Could you check a few things on this model? Use its own coordinates, in mm. Face numbers are marked on the shaded views. A direction names the side the tool comes from. Give positions to 0.01 mm unless a question says otherwise; leave off trailing zeros. Order: outer loops, then holes, each group sorted by start corner. A loop starts at its lowest first (then second) coordinate and runs counter-clockwise, first axis right, second up.
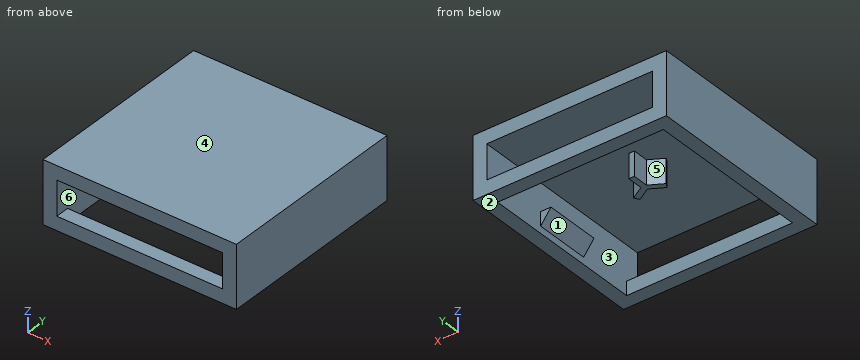
from build123d import *

# Parameters (mm, degrees)
SKETCH_1_W          = 28
SKETCH_1_H          = 28
EXTRUDE_1_DEPTH     = 2
SKETCH_2_W          = 28
SKETCH_2_H          = 28
SKETCH_2_W_2        = 24
SKETCH_2_H_2        = 24
EXTRUDE_2_DEPTH     = 7
SKETCH_3_W          = 24
SKETCH_3_H          = 5
CUT_EXTRUDE_1_DEPTH = 33.078029865
EXTRUDE_3_DEPTH     = 3.5
EXTRUDE_4_DEPTH     = 4


with BuildPart() as part:
    # Эскиз1 → Бобышка-Вытянуть1 (new body)
    with BuildSketch(Plane.XY):
        Rectangle(SKETCH_1_W, SKETCH_1_H)
    extrude(amount=EXTRUDE_1_DEPTH)

    # Эскиз2 → Бобышка-Вытянуть2 (add)
    with BuildSketch(Plane(origin=(0, 0, 0), x_dir=(-1, 0, 0), z_dir=(0, 0, -1))):
        Rectangle(SKETCH_2_W, SKETCH_2_H)
        Rectangle(SKETCH_2_W_2, SKETCH_2_H_2, mode=Mode.SUBTRACT)
    extrude(amount=EXTRUDE_2_DEPTH)

    # Эскиз3 → Вырез-Вытянуть1 (cut, through all)
    with BuildSketch(Plane(origin=(0, 14, 0), x_dir=(1, 0, 0), z_dir=(0, 1, 0))):
        with Locations((0, 2.5)):
            Rectangle(SKETCH_3_W, SKETCH_3_H)
    extrude(amount=-CUT_EXTRUDE_1_DEPTH, mode=Mode.SUBTRACT)

    # Эскиз4 → Бобышка-Вытянуть3 (add)
    with BuildSketch(Plane(origin=(0, 0, 0), x_dir=(-1, 0, 0), z_dir=(0, 0, -1))):
        with BuildLine():
            Line((-1.965063509, -1.596410162), (0, -0.461880215))
            Line((0, -0.461880215), (-0.2, -0.346410162))
            ThreePointArc((-0.2, -0.346410162), (-0.346410162, -0.2), (-0.4, 0))
            Line((-0.4, 0), (-0.4, 0.230940108))
            Line((-0.4, 0.230940108), (-2.365063509, -0.903589838))
            Line((-2.365063509, -0.903589838), (-1.965063509, -1.596410162))
        make_face()
        with BuildLine():
            Line((0, -0.461880215), (1.965063509, -1.596410162))
            Line((1.965063509, -1.596410162), (2.365063509, -0.903589838))
            Line((2.365063509, -0.903589838), (0.4, 0.230940108))
            Line((0.4, 0.230940108), (0.4, 0))
            ThreePointArc((0.4, 0), (0.346410162, -0.2), (0.2, -0.346410162))
            Line((0.2, -0.346410162), (0, -0.461880215))
        make_face()
        with BuildLine():
            Line((0.2, 0.346410162), (0.4, 0.230940108))
            Line((0.4, 0.230940108), (0.4, 2.5))
            Line((0.4, 2.5), (-0.4, 2.5))
            Line((-0.4, 2.5), (-0.4, 0.230940108))
            Line((-0.4, 0.230940108), (-0.2, 0.346410162))
            ThreePointArc((-0.2, 0.346410162), (0, 0.4), (0.2, 0.346410162))
        make_face()
        with BuildLine():
            Line((0, 0), (-0.2, -0.346410162))
            ThreePointArc((-0.2, -0.346410162), (0, -0.4), (0.2, -0.346410162))
            Line((0.2, -0.346410162), (0, 0))
        make_face()
        with BuildLine():
            Line((-0.2, 0.346410162), (0, 0))
            Line((0, 0), (0.2, 0.346410162))
            ThreePointArc((0.2, 0.346410162), (0, 0.4), (-0.2, 0.346410162))
        make_face()
        with BuildLine():
            Line((0, 0), (0.2, -0.346410162))
            ThreePointArc((0.2, -0.346410162), (0.346410162, -0.2), (0.4, 0))
            Line((0.4, 0), (0, 0))
        make_face()
        with BuildLine():
            Line((-0.4, 0), (0, 0))
            Line((0, 0), (-0.2, 0.346410162))
            ThreePointArc((-0.2, 0.346410162), (-0.346410162, 0.2), (-0.4, 0))
        make_face()
        with BuildLine():
            ThreePointArc((-0.4, 0), (-0.346410162, -0.2), (-0.2, -0.346410162))
            Line((-0.2, -0.346410162), (0, 0))
            Line((0, 0), (-0.4, 0))
        make_face()
        with BuildLine():
            Line((0.2, 0.346410162), (0, 0))
            Line((0, 0), (0.4, 0))
            ThreePointArc((0.4, 0), (0.346410162, 0.2), (0.2, 0.346410162))
        make_face()
        with BuildLine():
            Line((-0.2, -0.346410162), (0, -0.461880215))
            Line((0, -0.461880215), (0.2, -0.346410162))
            ThreePointArc((0.2, -0.346410162), (0, -0.4), (-0.2, -0.346410162))
        make_face()
        with BuildLine():
            Line((0.4, 0), (0.4, 0.230940108))
            Line((0.4, 0.230940108), (0.2, 0.346410162))
            ThreePointArc((0.2, 0.346410162), (0.346410162, 0.2), (0.4, 0))
        make_face()
        with BuildLine():
            Line((-0.4, 0.230940108), (-0.4, 0))
            ThreePointArc((-0.4, 0), (-0.346410162, 0.2), (-0.2, 0.346410162))
            Line((-0.2, 0.346410162), (-0.4, 0.230940108))
        make_face()
    extrude(amount=EXTRUDE_3_DEPTH)

    # Эскиз6 → Бобышка-Вытянуть4 (add, symmetric)
    with BuildSketch(Plane(origin=(0, 0, 0), x_dir=(1, 0, 0), z_dir=(0, 1, 0))):
        Polygon((-12, 6), (-10.5, 4), (-12, 4), align=None)
    extrude_4 = extrude(amount=EXTRUDE_4_DEPTH, both=True)

    # Зеркальное отражение1: Бобышка-Вытянуть4 across plane
    add(extrude_4.mirror(Plane(origin=(0, 0, 0), x_dir=(0, 0, 1), z_dir=(1, 0, 0))))


solid = part.part
Item 1: Please list where these lines run through material, in increasing order: line 1 along X through (y, z) = (-7.25, -5.75); line 2 along Z through (x, y) = (7.75, -11.75).
Findings:
line 1: x = -14 to -12, 12 to 14
line 2: z = 0 to 2
Item 2: We'd pull the mould along Y, two halves only. Please class the marked faces 4, 5 and 6: +Y half, -Y half, draft (parallel to the pull), parting line (faces both ways), or undercut.
Findings:
face 4: draft
face 5: +Y half
face 6: undercut
Item 3: Imagine slicing it at A-A on x = -3. List the corners of the cut face in (y, z) for me.
Findings:
outline: (-14, -7) - (-12, -7) - (-12, -5) - (-14, -5) - close; (-14, 0) - (14, 0) - (14, 2) - (-14, 2) - close; (12, -7) - (14, -7) - (14, -5) - (12, -5) - close
Item 4: Imagine slicing it at B-B on z = -0.5. List the corners of the cut face in (x, y) for me, then the cut area to 3 significant figures.
Findings:
outline: (-14, -14) - (-12, -14) - (-12, 14) - (-14, 14) - close; (-2.37, -0.9) - (-1.97, -1.6) - (0, -0.46) - (1.97, -1.6) - (2.37, -0.9) - (0.4, 0.23) - (0.4, 2.5) - (-0.4, 2.5) - (-0.4, 0.23) - close; (12, -14) - (14, -14) - (14, 14) - (12, 14) - close
area: 118 mm2
Item 5: Imagine slicing it at D-D on x = -11.5. List the corners of the cut face in (y, z) for me.
Findings:
outline: (-14, -7) - (-12, -7) - (-12, -5) - (-14, -5) - close; (-14, 0) - (14, 0) - (14, 2) - (-14, 2) - close; (-4, -5.33) - (4, -5.33) - (4, -4) - (-4, -4) - close; (12, -7) - (14, -7) - (14, -5) - (12, -5) - close
Item 6: For the marked faces 1, 2 and 3, which set-ups out of +Z, -Z, +X, -X, +Y, -Y let a thin tool reach every point of the face, with its end or its side?
Findings:
face 1: -Z
face 2: -Z, +X, -X, +Y, -Y
face 3: none
Item 7: Imagine slicing it at C-C on y = 3.5. List the corners of the cut face in (x, z) for me, then the cut area to 3 significant figures.
Findings:
outline: (-14, -7) - (-12, -7) - (-12, -6) - (-10.5, -4) - (-12, -4) - (-12, 0) - (12, 0) - (12, -4) - (10.5, -4) - (12, -6) - (12, -7) - (14, -7) - (14, 2) - (-14, 2) - close
area: 87.0 mm2
Item 8: For pin 1 (3 mm diameter, centred on x = 7.5, y = 5.5, fed in from -Z); pin 2 (1.2 mm diameter, centred on x = 1, y = 0, fed in from -Z), each with a flat end and sliding along its axis, tell me the tip position at first contact or that it passes through.
Findings:
pin 1: stops at z = 0
pin 2: stops at z = -3.5
